Can you work these out from the model? Positions are in its coordinate system, mm. A direction names the side the tool comes from. Give positions to 0.01 mm unless a question says otherwise; leave off trailing zeros. Loops run counter-clockwise (first coordinate to the right, second up) from the corner with the lowest first, then second, coordinate; pieces in that order, holes last.
from build123d import *

# Parameters (mm, degrees)
ESQUISSE1_R             = 31.75
BOSS_EXTRU_1_DEPTH      = 50.8
ESQUISSE3_W             = 4.13004
ESQUISSE3_H             = 63.5
ENL_V_MAT_EXTRU_1_DEPTH = 44.45


with BuildPart() as part:
    # Esquisse1 → Boss.-Extru.1 (new body)
    with BuildSketch(Plane.XY):
        Circle(ESQUISSE1_R)
    extrude(amount=BOSS_EXTRU_1_DEPTH)

    # Esquisse3 → Enlèv. mat.-Extru.1 (cut)
    with BuildSketch(Plane(origin=(0, 0, 0), x_dir=(-1, 0, 0), z_dir=(0, 0, -1))):
        with Locations((-16.96212, 0)):
            Rectangle(ESQUISSE3_W, ESQUISSE3_H)
        with Locations((-25.34412, 0)):
            Rectangle(ESQUISSE3_W, ESQUISSE3_H)
        with Locations((-8.58012, 0)):
            Rectangle(ESQUISSE3_W, ESQUISSE3_H)
        with Locations((-0.19812, 0)):
            Rectangle(ESQUISSE3_W, ESQUISSE3_H)
        with Locations((8.18388, 0)):
            Rectangle(ESQUISSE3_W, ESQUISSE3_H)
        with Locations((16.56588, 0)):
            Rectangle(ESQUISSE3_W, ESQUISSE3_H)
        with Locations((24.94788, 0)):
            Rectangle(ESQUISSE3_W, ESQUISSE3_H)
    extrude(amount=-ENL_V_MAT_EXTRU_1_DEPTH, mode=Mode.SUBTRACT)


solid = part.part
(1) Suppose I cut it at C-C on x = 0. List the corners of the cut face in (y, z) for me.
Returned:
outline: (-31.75, 44.45) - (31.75, 44.45) - (31.75, 50.8) - (-31.75, 50.8) - close
(2) Which directions (+Z, -Z, +X, -X, +Y, -Y) give clear straight access to the entire face, cutting with the end or side of a thin tool? Please do faces 5 (the flat face through (-22.883, 0, 22)), 6 (the flat face through (29, 0, 0)).
Returned:
face 5: -Z, +Y, -Y
face 6: -Z, +X, -X, +Y, -Y
(3) Suppose I cut it at A-A on z = 5.5. List the corners of the cut face in (x, y) for me, plus the area to 3 significant figures.
Returned:
outline: (-27.01, -16.68) - (-27.01, 16.68) arc R31.75 ccw to start; (-22.88, -22.01) arc R31.75 ccw to (-18.63, -25.71) - (-18.63, 25.71) arc R31.75 ccw to (-22.88, 22.01) - close; (-14.5, -28.25) arc R31.75 ccw to (-10.25, -30.05) - (-10.25, 30.05) arc R31.75 ccw to (-14.5, 28.25) - close; (-6.12, -31.15) arc R31.75 ccw to (-1.87, -31.7) - (-1.87, 31.7) arc R31.75 ccw to (-6.12, 31.15) - close; (2.26, -31.67) arc R31.75 ccw to (6.52, -31.07) - (6.52, 31.07) arc R31.75 ccw to (2.26, 31.67) - close; (10.65, -29.91) arc R31.75 ccw to (14.9, -28.04) - (14.9, 28.04) arc R31.75 ccw to (10.65, 29.91) - close; (19.03, -25.42) arc R31.75 ccw to (23.28, -21.59) - (23.28, 21.59) arc R31.75 ccw to (19.03, 25.42) - close; (27.41, -16.03) arc R31.75 ccw to (27.41, 16.03) - close
area: 1,640 mm2
(4) Suppose I cut it at D-D on y = -20. List the corners of the cut face in (x, z) for me.
Returned:
outline: (-24.66, 44.45) - (-22.88, 44.45) - (-22.88, 0) - (-18.63, 0) - (-18.63, 44.45) - (-14.5, 44.45) - (-14.5, 0) - (-10.25, 0) - (-10.25, 44.45) - (-6.12, 44.45) - (-6.12, 0) - (-1.87, 0) - (-1.87, 44.45) - (2.26, 44.45) - (2.26, 0) - (6.52, 0) - (6.52, 44.45) - (10.65, 44.45) - (10.65, 0) - (14.9, 0) - (14.9, 44.45) - (19.03, 44.45) - (19.03, 0) - (23.28, 0) - (23.28, 44.45) - (24.66, 44.45) - (24.66, 50.8) - (-24.66, 50.8) - close
(5) Will these pins go through, and if not, where does the flat tip stop? P1, Ø22, axis at y = 12, z = 18.5, coming from the -X side; P2, Ø22, axis at y = 15, z = 31.5, coming from the -X side; P3, Ø2, axis at x = 23, z = 14, coming from the +Y side.
Returned:
P1: stops at x = -31.73
P2: stops at x = -31.5
P3: stops at y = 22.89
(6) Please list where these lines run through material, in increasing order: probe 1 along X at (y, z) = (21, 39); probe 2 along X at (y, z) = (-28, 42.5); probe 3 along X at (y, z) = (25.5, 9).
Returned:
probe 1: x = -22.88 to -18.63, -14.5 to -10.25, -6.12 to -1.87, 2.26 to 6.52, 10.65 to 14.9, 19.03 to 23.28
probe 2: x = -14.5 to -10.25, -6.12 to -1.87, 2.26 to 6.52, 10.65 to 14.9
probe 3: x = -18.92 to -18.63, -14.5 to -10.25, -6.12 to -1.87, 2.26 to 6.52, 10.65 to 14.9
(7) Thinking about a two-plate mould opening in X: for faces 1 (the flat face through (-8, 0, 44.45)), 2 (the cylindrical face through (30.284, 9.537, 25.044)), 3 (the flat face through (-6.119, 0, 22)), 4 (the flat face through (13, 0, 0)), which applies, pulls with the +X half, pulls with the -X half, needs draft (parallel to the pull), parting line crosses it, or undercut?
Returned:
face 1: undercut
face 2: parting line crosses it
face 3: undercut
face 4: needs draft
